from build123d import *

# Parameters (mm, degrees)
ESQUISSE1_R                  = 30.5
EXTRUSION1_DEPTH             = 1
ENL_V_MAT_EXTRU_1_DEPTH      = 2
R_P_TITION_CIRCULAIRE1_COUNT = 15
ESQUISSE3_R                  = 21
EXTRUSION2_DEPTH             = 2.125
ESQUISSE4_R                  = 16
ENL_V_MAT_EXTRU_2_DEPTH      = 3.125
ENL_V_MAT_EXTRU_2_DEPTH_BACK = 3.125
CHANFREIN1_SIZE              = 0.5


with BuildPart() as part:
    # Esquisse1 → Extrusion1 (new body, symmetric)
    with BuildSketch(Plane.XY):
        Circle(ESQUISSE1_R)
    extrude(amount=EXTRUSION1_DEPTH, both=True)

    # Esquisse2 → Enlèv. mat.-Extru.1 (cut, symmetric)
    with BuildSketch(Plane.XY):
        with BuildLine():
            Line((-5.262955088, 30.042491637), (-3.276608177, 27.205694255))
            ThreePointArc((-3.276608177, 27.205694255), (0.940808513, 25.612214082), (3.963058372, 28.957627119))
            Line((3.963058372, 28.957627119), (4.13559322, 30.218320084))
            ThreePointArc((4.13559322, 30.218320084), (-0.570495492, 30.49466404), (-5.262955088, 30.042491637))
        make_face()
    enl_v_mat_extru_1 = extrude(amount=ENL_V_MAT_EXTRU_1_DEPTH, both=True, mode=Mode.SUBTRACT)

    # Répétition circulaire1: Enlèv. mat.-Extru.1 ×15 about axis
    r_p_tition_circulaire1_axis = Axis((0, 0, 0), (0, 0, 1))
    for i in range(1, R_P_TITION_CIRCULAIRE1_COUNT):
        add(enl_v_mat_extru_1.rotate(r_p_tition_circulaire1_axis, i * 360 / R_P_TITION_CIRCULAIRE1_COUNT), mode=Mode.SUBTRACT)

    # Esquisse3 → Extrusion2 (add, symmetric)
    with BuildSketch(Plane.XY):
        Circle(ESQUISSE3_R)
    extrude(amount=EXTRUSION2_DEPTH, both=True)

    # Esquisse4 → Enlèv. mat.-Extru.2 (cut, two sides)
    with BuildSketch(Plane.XY) as enl_v_mat_extru_2_sk:
        Circle(ESQUISSE4_R)
    extrude(amount=ENL_V_MAT_EXTRU_2_DEPTH, mode=Mode.SUBTRACT)
    extrude(enl_v_mat_extru_2_sk.sketch, amount=-ENL_V_MAT_EXTRU_2_DEPTH_BACK, mode=Mode.SUBTRACT)

    # Chanfrein1
    chanfrein1_edges = [part.edges().sort_by_distance(p)[0] for p in [
        (-21, 0, -2.125),
        (-21, 0, 2.125),
        (-16, 0, -2.125),
        (-16, 0, 2.125),
    ]]
    chamfer(chanfrein1_edges, length=CHANFREIN1_SIZE)


solid = part.part
Verification items for the finished model (mm, model axes). A direction names the side the tool comes from. Coordinates: 2 decimals unless noted, no trailing zeros. Order: outer loops, then holes, each group sorted by start corner. A loop starts at its lowest first (then second) coordinate and runs counter-clockwise, first axis right, second up.
1. Set-up check for faces 5 (the face through (18.42, 22.35, 0.01)), 6 (the face through (10.15, -27.13, 0.01)), 7 (the face through (14.34, -21.22, 0.01)), 8 (the face through (-15.564, 24.425, 0.014)): record each of +Z, -Z, +X, -X, +Y, -Y from which the full face is reachable in a straight line by a thin tool's end or side.
Results found:
face 5: +Z, -Z, +X
face 6: +Z, -Z, -Y
face 7: +Z, -Z
face 8: +Z, -Z, +Y
2. Go/stop test with flat-tipped pins: pin 1 Ø2 at (y, z) = (-22, 1) entering from -X; pin 2 Ø3 at (x, y) = (-7, 24) entering from -Z; pin 3 Ø1.5 at (y, z) = (16.5, 1) entering from +X. Record where each tip stops, or that it passes through.
Results found:
pin 1: stops at x = -22.12
pin 2: stops at z = -1
pin 3: stops at x = 26.12
3. Sectioned sample at A-A, the plane x = 0. Record the cut outline in (y, z) (3 decimals).
Results found:
outline: (-30.5, -1) - (-21, -1) - (-21, -1.625) - (-20.5, -2.125) - (-16.5, -2.125) - (-16, -1.625) - (-16, 1.625) - (-16.5, 2.125) - (-20.5, 2.125) - (-21, 1.625) - (-21, 1) - (-30.5, 1) - close; (16, -1.625) - (16.5, -2.125) - (20.5, -2.125) - (21, -1.625) - (21, -1) - (25.5, -1) - (25.5, 1) - (21, 1) - (21, 1.625) - (20.5, 2.125) - (16.5, 2.125) - (16, 1.625) - close
4. Release check for a two-part mould opening along X. For faces 1 (the face through (20.03, 6.31, -1.31)), 2 (the face through (-3.47, -15.62, 0.02)), 3 (the face through (-11.904, -28.081, 0.014)), 4 (the face through (21.73, -13.56, 0.01)) record: +X half, -X half, draft (parallel to the pull), parting line (faces both ways), or undercut.
Results found:
face 1: parting line
face 2: undercut
face 3: -X half
face 4: +X half
5. Scan lines: line 1 (Y direction, x = 0, z = 0.7); line 2 (Z direction, x = 2, y = 25.5); line 3 (X direction, y = 0, z = -0.3). Record each from-to range of solid material in increasing order.
Results found:
line 1: y = -30.5 to -16, 16 to 25.5
line 2: z = -1 to 1
line 3: x = -26.79 to -16, 16 to 26.79
